The listing builds one solid part. Answer for the finished solid, in the listing's coordinates (mm). Face numbers are marked on the shaded views. Give positions to 0.01 mm unless a question says otherwise; leave off trailing zeros. Write each loop counter-clockwise with the first axis right and the second up, starting at its lowest first coordinate (ties: lowest second). Pieces come first, ordered by that corner, then holes. Notation, with made-up numbers: (13.25, 3) -> (45.25, 3) arc R22 cw to (45.25, 9) -> close; hole circle Ø7 at (-8, 54.25). An arc over 180 degrees is marked (long way). Write each question's results on one line, items separated by ' | '. Start each with the question number.
from build123d import *

# Parameters (mm, degrees)
BOSS_EXTRUDE1_DEPTH = 200
CHAMFER1_SIZE       = 130
CHAMFER1_SIZE2      = 170
CHAMFER2_SIZE       = 170
CHAMFER2_SIZE2      = 130
FILLET1_R           = 50
SKETCH2_R           = 20
BOSS_EXTRUDE2_DEPTH = 10


with BuildPart() as part:
    # Sketch1 → Boss-Extrude1 (new body)
    with BuildSketch(Plane.XY):
        with BuildLine():
            Line((0, 0), (-300, 0))
            Line((-300, 0), (-335.355339059, 35.355339059))
            Line((-335.355339059, 35.355339059), (-300, 70.710678119))
            ThreePointArc((-300, 70.710678119), (-174.539840649, 100.365711492), (-49.079681299, 70.710678119))
            ThreePointArc((-49.079681299, 70.710678119), (-18.96069104, 74.015201956), (0, 97.649195424))
            ThreePointArc((0, 97.649195424), (36.003553141, 223.252657901), (132.842160393, 310.972494714))
            ThreePointArc((132.842160393, 310.972494714), (161.131495087, 329.380753651), (168.11847076, 362.400938773))
            Line((168.11847076, 362.400938773), (168.11847076, 567.864757456))
            Line((168.11847076, 567.864757456), (198.11847076, 567.864757456))
            Line((198.11847076, 567.864757456), (198.11847076, 343.151257275))
            Line((198.11847076, 343.151257275), (0, 0))
        make_face()
    extrude(amount=-BOSS_EXTRUDE1_DEPTH)

    # Mirror1: part across plane


with BuildPart() as part_1:
    add(part.part)
    add(part.part.mirror(Plane(origin=(-174.539840649, -179.851012248, -200), x_dir=(1, 0, 0), z_dir=(0, 0, -1))))

    # Chamfer1
    chamfer1_edges = [part_1.edges().sort_by_distance(p)[0] for p in [
        (183.11847076, 567.864757456, 0),
    ]]
    chamfer1_side = [part_1.faces().sort_by_distance(p)[0] for p in [
        (183.11847076, 567.864757456, -200),
    ]]
    chamfer(chamfer1_edges, length=CHAMFER1_SIZE, length2=CHAMFER1_SIZE2, reference=chamfer1_side[0])

    # Chamfer2
    chamfer2_edges = [part_1.edges().sort_by_distance(p)[0] for p in [
        (183.11847076, 567.864757456, -400),
    ]]
    chamfer2_side = [part_1.faces().sort_by_distance(p)[0] for p in [
        (190.327035151, 455.508007366, -400),
    ]]
    chamfer(chamfer2_edges, length=CHAMFER2_SIZE, length2=CHAMFER2_SIZE2, reference=chamfer2_side[0])

    # Fillet1
    fillet1_edges = [part_1.edges().sort_by_distance(p)[0] for p in [
        (183.11847076, 397.864757456, 0),
        (183.11847076, 567.864757456, -130),
        (183.11847076, 567.864757456, -270),
        (183.11847076, 397.864757456, -400),
    ]]
    fillet(fillet1_edges, radius=FILLET1_R)

    # Sketch2 → Boss-Extrude2 (add)
    with BuildSketch(Plane.XZ):
        with Locations((-150, -200)):
            Circle(SKETCH2_R)
    extrude(amount=BOSS_EXTRUDE2_DEPTH)


solid = part_1.part
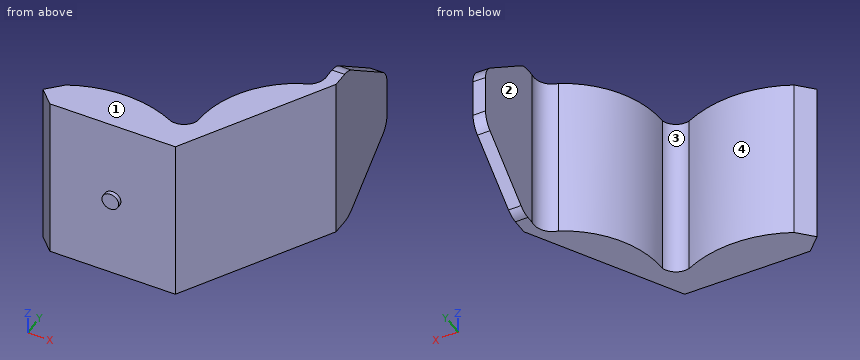
1. Consider probe 1 along X at (y, z) = (367, -158); probe 2 along Y at (x, z) = (-169, -366); probe 3 along Y at (x, z) = (-295, -368). Determine where each line is inside the solid, lowest interval first. Write a range as [from, to].
2. Section C-C (y = 397.5) is taken. Write down the section's boundary in (x, z), then the cut area to 3 significant figures.
3. Section D-D (z = -85) is taken. Write down the section's boundary in (x, y), then the cut area to 3 significant figures.
4. The mould has two halves that part along X. Classify the marked faces 1, 2, 3 and 4: pulls with the +X half, pulls with the -X half, needs draft (parallel to the pull), parting line crosses it, or undercut.
5. Each of these flat-tipped pins is pushed along its axis until it touches: pin 1 Ø12 at (y, z) = (240.5, -255) entering from -X; pin 2 Ø5 at (y, z) = (244, -298.5) entering from -X; pin 3 Ø3 at (x, z) = (140, -230) entering from +Y (3 decimals). Where does it stop, or does it pass through?
6. Section A-A (z = -200) is taken. Write down the section's boundary in (x, y).
7. Section B-B (x = -150) is taken. Write down the section's boundary in (y, z).
Results:
1) probe 1: x = [168.12, 198.12] | probe 2: y = [0, 100.31] | probe 3: y = [0, 73.15]
2) outline: (168.12, -397.18) -> (198.12, -397.18) -> (198.12, -2.82) -> (168.12, -2.82) -> close | area: 11,800 mm²
3) outline: (-335.36, 35.36) -> (-300, 0) -> (0, 0) -> (198.12, 343.15) -> (198.12, 509.02) -> (168.12, 509.02) -> (168.12, 362.4) arc R44.1 cw to (132.84, 310.97) arc R238.22 ccw to (0, 97.65) arc R39.59 cw to (-49.08, 70.71) arc R280.22 ccw to (-300, 70.71) -> close | area: 53,500 mm²
4) face 1: needs draft | face 2: pulls with the -X half | face 3: undercut | face 4: undercut
5) pin 1: stops at x = 43.46 | pin 2: stops at x = 48.58 | pin 3: stops at y = 313.525
6) outline: (-335.36, 35.36) -> (-300, 0) -> (-170, 0) -> (-170, -10) -> (-130, -10) -> (-130, 0) -> (0, 0) -> (198.12, 343.15) -> (198.12, 567.86) -> (168.12, 567.86) -> (168.12, 362.4) arc R44.1 cw to (132.84, 310.97) arc R238.22 ccw to (0, 97.65) arc R39.59 cw to (-49.08, 70.71) arc R280.22 ccw to (-300, 70.71) -> close
7) outline: (-10, -220) -> (0, -220) -> (0, -400) -> (99.29, -400) -> (99.29, 0) -> (0, 0) -> (0, -180) -> (-10, -180) -> close
